from build123d import *

# Parameters (mm, degrees)
BOSS_EXTRUDE1_DEPTH = 17
BOSS_EXTRUDE2_DEPTH = 10
SKETCH3_R           = 5
CUT_EXTRUDE1_DEPTH  = 17
BOSS_EXTRUDE3_DEPTH = 13


with BuildPart() as part:
    # Sketch1 → Boss-Extrude1 (new body)
    with BuildSketch(Plane.XY):
        Polygon((-35.219488433, -14.864106981), (-4.219488433, -14.864106981), (-4.219488433, -4.864106981), (31.780511567, -4.864106981), (31.780511567, -14.864106981), (62.780511567, -14.864106981), (30.780511567, 15.135893019), (20.780511567, 15.135893019), (4.780511567, 15.135893019), (-5.219488433, 15.135893019), align=None)
    extrude(amount=-BOSS_EXTRUDE1_DEPTH)

    # Sketch2 → Boss-Extrude2 (add)
    with BuildSketch(Plane.XY):
        with BuildLine():
            ThreePointArc((22.780511567, 15.135893019), (12.780511567, 25.135893019), (2.780511567, 15.135893019))
            Line((2.780511567, 15.135893019), (22.780511567, 15.135893019))
        make_face()
        with BuildLine():
            Line((22.780511567, 15.135893019), (2.780511567, 15.135893019))
            ThreePointArc((2.780511567, 15.135893019), (12.780511567, 5.135893019), (22.780511567, 15.135893019))
        make_face()
    extrude(amount=-BOSS_EXTRUDE2_DEPTH)

    # Sketch3 → Cut-Extrude1 (cut)
    with BuildSketch(Plane.XY):
        with Locations((12.780511567, 15.135893019)):
            Circle(SKETCH3_R)
    extrude(amount=-CUT_EXTRUDE1_DEPTH, mode=Mode.SUBTRACT)

    # Sketch4 → Boss-Extrude3 (add)
    with BuildSketch(Plane(origin=(0, 0, -17), x_dir=(-1, 0, 0), z_dir=(0, 0, -1))):
        Polygon((-62.780511567, -14.864106981), (-45.7138449, 1.135893019), (19.219488433, 1.135893019), (35.219488433, -14.864106981), (4.219488433, -14.864106981), (4.219488433, -4.864106981), (-31.780511567, -4.864106981), (-31.780511567, -14.864106981), align=None)
    extrude(amount=BOSS_EXTRUDE3_DEPTH)

    # Mirror9: part across plane


with BuildPart() as part_1:
    add(part.part)
    add(part.part.mirror(Plane(origin=(0, 0, -30), x_dir=(1, 0, 0), z_dir=(0, 0, -1))))


solid = part_1.part
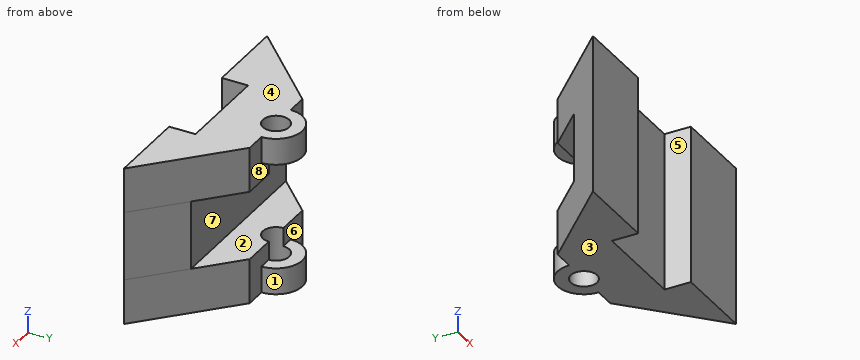
The listing builds one solid part. Answer for the finished solid, in the listing's coordinates (mm). Face numbers are marked on the shaded views. A direction names the side the tool comes from. Coordinates: 2 decimals unless noted, no trailing zeros. Loops run counter-clockwise (first coordinate to the right, second up) from the corner with the lowest first, then second, coordinate; pieces in that order, holes last. Notation, with made-up numbers: (-30.5, 48.5) -> (27.5, 48.5) arc R17 ccw to (27.5, 80.5) -> close; hole circle Ø10 at (-23, 1). An arc over 180 degrees is marked (long way). Answer in a Markdown table with one row per item. Add a question column.
1. The part is cut by section C-C, the plane y = 17.5. Write down the section's boundary in (x, z).
2. For the marked faces 5, 6, 7 and 8, determine the directions among +Z, -Z, +X, -X, +Y, -Y from which every point of the face is accessible in a straight line to the end or side of a thin tool.
3. Flat-ended cylindrical pins translate along their axes: P1, Ø12, axis at x = 38, z = -46.5, coming from the +Y side; P2, Ø1, axis at x = 0.5, z = -22.5, coming from the -Y side; P3, Ø11, axis at y = -9, z = -16.5, coming from the +X side. Find the tip coordinate at first contact, or state that the pin passes through.
4. The part is cut by section D-D, the plane z = -16. Write down the section's boundary in (x, y).
5. The part is cut by section B-B, the plane y = 4. Write down the section's boundary in (x, z).
6. Determine the mould class of the marked faces 1, 2, 3 and 4 for opening direction Z: +Z half, -Z half, draft (parallel to the pull), parting line (faces both ways), or undercut.
7. The part is cut by section A-A, the plane z = -6. Write down the section's boundary in (x, y).
8. Consider line 1 (Z direction, x = -7.5, y = 2); line 2 (Z direction, x = 10, y = 23); line 3 (Y direction, x = -4, z = -41). Determine where each line is inside the solid, lowest interval first. Write a range as [from, to].
Answer below:
| question | item | result |
|---|---|---|
| 1 | outline | (3.06, -60) -> (8.37, -60) -> (8.37, -50) -> (3.06, -50) -> close; (3.06, -10) -> (8.37, -10) -> (8.37, 0) -> (3.06, 0) -> close; (17.19, -60) -> (22.5, -60) -> (22.5, -50) -> (17.19, -50) -> close; (17.19, -10) -> (22.5, -10) -> (22.5, 0) -> (17.19, 0) -> close |
| 2 | face 5 | +Z, -Z, -Y |
| 2 | face 6 | -X, +Y |
| 2 | face 7 | +X, -X, +Y |
| 2 | face 8 | +X, +Y |
| 3 | P1 | y = 13.99 |
| 3 | P2 | y = -4.86 |
| 3 | P3 | x = 62.39 |
| 4 | outline | (-35.22, -14.86) -> (-4.22, -14.86) -> (-4.22, -4.86) -> (31.78, -4.86) -> (31.78, -14.86) -> (62.78, -14.86) -> (30.78, 15.14) -> (17.78, 15.14) arc R5 cw to (7.78, 15.14) -> (-5.22, 15.14) -> close |
| 5 | outline | (-16.36, -60) -> (42.66, -60) -> (42.66, -43) -> (-16.36, -43) -> close; (-16.36, -17) -> (42.66, -17) -> (42.66, 0) -> (-16.36, 0) -> close |
| 6 | face 1 | draft |
| 6 | face 2 | undercut |
| 6 | face 3 | -Z half |
| 6 | face 4 | +Z half |
| 7 | outline | (-35.22, -14.86) -> (-4.22, -14.86) -> (-4.22, -4.86) -> (31.78, -4.86) -> (31.78, -14.86) -> (62.78, -14.86) -> (30.78, 15.14) -> (22.78, 15.14) arc R10 ccw to (2.78, 15.14) -> (-5.22, 15.14) -> close; hole circle Ø10 at (12.78, 15.14) |
| 8 | line 1 | [-60, -43], [-17, 0] |
| 8 | line 2 | [-60, -50], [-10, 0] |
| 8 | line 3 | [-4.86, 1.14] |
